from build123d import *

# Parameters (mm, degrees)
F0_W     = 76.2
F0_H     = 50.8
F1_DEPTH = 6.35
F3_W     = 50.8
F3_H     = 63.5
F4_DEPTH = 6.35
F5_R     = 2.5


with BuildPart() as f1:
    # F0 (on Top) → F1 (new body)
    with BuildSketch(Plane.XY):
        with Locations((1.0298034176, -8.9605891951)):
            Rectangle(F0_W, F0_H)
    extrude(amount=F1_DEPTH)

    # F3 (on offset) → F4 (join)
    with BuildSketch(Plane.YZ.offset(21)):
        with Locations((-8.8295020819, -31.75)):
            Rectangle(F3_W, F3_H)
    extrude(amount=F4_DEPTH)

    # F5
    f5_edges = [f1.edges().sort_by_distance(p)[0] for p in [
        (21, -8.895046, 0),
        (27.35, -8.895046, 0),
    ]]
    fillet(f5_edges, radius=F5_R)


solid = f1.part
Part model, mm, in its own coordinate system. A direction names the side the tool comes from. Round coordinates to 2 decimals unless told otherwise and drop trailing zeros. Write each loop counter-clockwise with the first axis right and the second up, starting at its lowest first coordinate (ties: lowest second). Pieces come first, ordered by that corner, then holes. Notation, with made-up numbers: M 11,9 L 17,9 A15 ccw 17,14 Z; hole C 54,12.5 d3. An arc over 180 degrees is marked long. Return JSON: item names as keys, results as strings. Group by question number.
(1) Saw through at C-C on x = 10.5. Write the cut outline in (y, z), then the cut area to 3 significant figures.
(2) Saw through at A-A on y = -15. Write the cut outline in (x, z).
(3) Drill centre lines: probe 1 along X at (y, z) = (-10, -6.5); probe 2 along Z at (x, y) = (-25.5, 10.5); probe 3 along Y at (x, z) = (26, -7.5). Where is each one in solid material? Low to high.
(4) Saw through at B-B on z = -20.5. Write the cut outline in (x, y), then the cut area to 3 significant figures.
(5) Which spindle directions (+Z, -Z, +X, -X, +Y, -Y) get a long thin tool onto all of the face, cutting with end or side? Do faces 1 (the face through (0, -9, 0)), 2 (the face through (21, -9, -31)), 3 (the face through (24, -34.23, -32)). Say none if no direction does.
(6) Pin check, flat tips, straight feed: pin 1 Ø1.5 at (y, z) = (-0.5, -44) entering from +X; pin 2 Ø1.5 at (x, y) = (-11.5, -1) entering from -Z; pin 3 Ø2.5 at (x, z) = (-11, 0) entering from +Y. Stop position of each tip, or through.
Returned:
{
 "1": {"outline": "M -34.36,0 L 16.44,0 L 16.44,6.35 L -34.36,6.35 Z", "area": "323 mm²"},
 "2": {"outline": "M -37.07,0 L 18.5,0 A2.5 cw 21,-2.5 L 21,-63.5 L 27.35,-63.5 L 27.35,-2.5 A2.5 cw 29.85,0 L 39.13,0 L 39.13,6.35 L -37.07,6.35 Z"},
 "3": {"probe 1": "21 to 27.35", "probe 2": "0 to 6.35", "probe 3": "-34.23 to 16.57"},
 "4": {"outline": "M 21,-34.23 L 27.35,-34.23 L 27.35,16.57 L 21,16.57 Z", "area": "323 mm²"},
 "5": {"face 1": "-Z, +Y, -Y", "face 2": "-Z, -X, +Y, -Y", "face 3": "-Z, +X, -X, -Y"},
 "6": {"pin 1": "x = 27.35", "pin 2": "z = 0", "pin 3": "y = 16.44"}
}
